Verification items for this drawing (mm, ordinates from the low corner). A direction names the side the tool comes from. Give positions to 0.01 mm unless a question says otherwise; leave off trailing zeros. Loops run counter-clockwise (first coordinate to the right, second up) from the corner with the lowest first, then second, coordinate; pieces in that order, holes last. Notation, with made-up numbers: M 10,-9.75 L 30,-9.75 A15 ccw 30,-4.75 Z; hole C -8,17 d7. An arc over 180 degrees is marked long. Use one line per item in the form item = value.
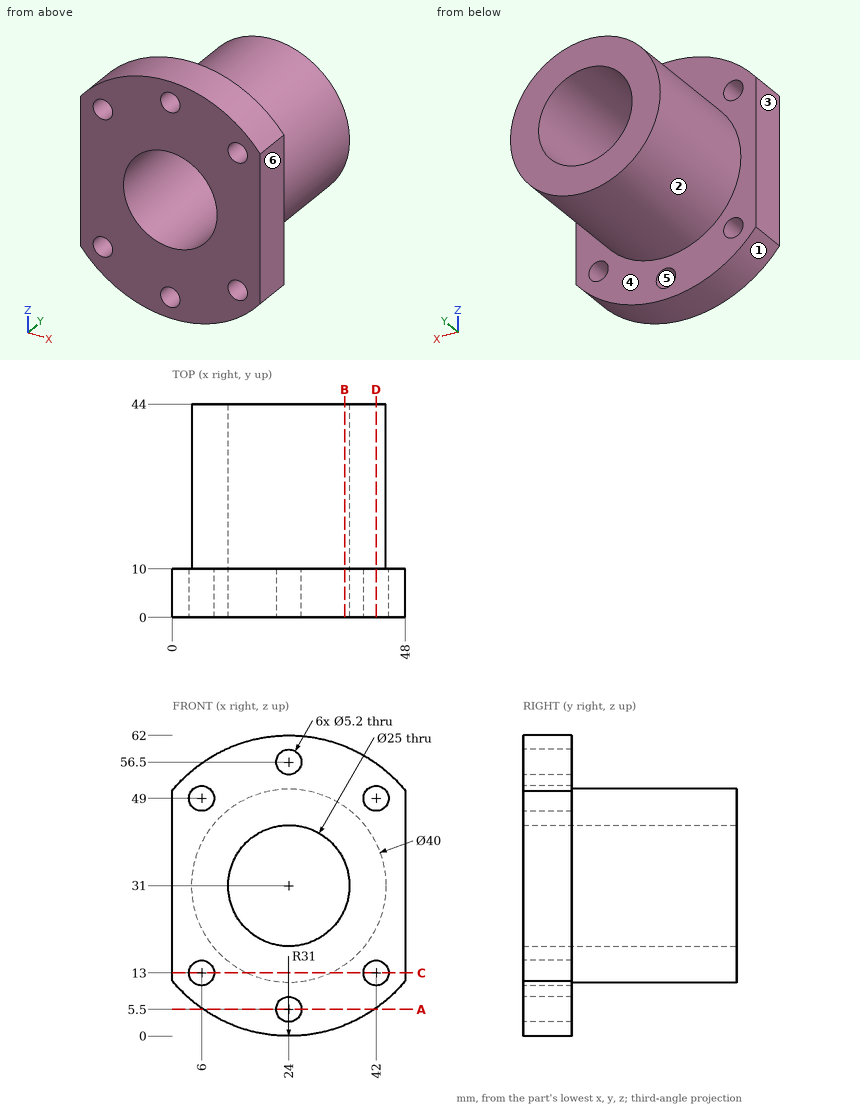
1) Section check C-C (z = 13). Record the cut outline in (x, y).
Evaluation:
outline = M 0,0 L 3.4,0 L 3.4,10 L 0,10 Z; M 8.6,0 L 39.4,0 L 39.4,10 L 32.72,10 L 32.72,44 L 15.28,44 L 15.28,10 L 8.6,10 Z; M 44.6,0 L 48,0 L 48,10 L 44.6,10 Z
2) Section check B-B (x = 35.5). Record the cut outline in (y, z), then the cut area to 3 significant figures.
Evaluation:
outline = M 0,2.21 L 10,2.21 L 10,14.64 L 44,14.64 L 44,26.1 L 0,26.1 Z; M 0,35.9 L 44,35.9 L 44,47.36 L 10,47.36 L 10,59.79 L 0,59.79 Z
area = 1,260 mm^2
3) Set-up check for the marked faces 1 and 2: record each of +Z, -Z, +X, -X, +Y, -Y from which the full face is reachable in a straight line by a thin tool's end or side.
Evaluation:
face_1 = -Z, +Y, -Y
face_2 = +Y
4) Depth check by flat-ended pin: pin 1 Ø4 at (x, z) = (37.5, 51) entering from +Y; pin 2 Ø5 at (x, y) = (37.5, 16.5) entering from +Z; pin 3 Ø12 at (y, z) = (22.5, 22) entering from +X. Enter the tip coordinate at first touch or a pass-through.
Evaluation:
pin_1 = 10
pin_2 = 47.7
pin_3 = 43.77
5) Scan lines: line 1 (X direction, y = 7.5, z = 49); line 2 (X direction, y = 18, z = 31); line 3 (Z direction, x = 24, y = 35). Record each from-to range of solid material in increasing order.
Evaluation:
line_1 = 0 to 3.4, 8.6 to 39.4, 44.6 to 48
line_2 = 4 to 11.5, 36.5 to 44
line_3 = 11 to 18.5, 43.5 to 51
6) Section check D-D (x = 42). Record the cut outline in (y, z).
Evaluation:
outline = M 0,5.76 L 10,5.76 L 10,10.4 L 0,10.4 Z; M 0,15.6 L 10,15.6 L 10,22.28 L 44,22.28 L 44,39.72 L 10,39.72 L 10,46.4 L 0,46.4 Z; M 0,51.6 L 10,51.6 L 10,56.24 L 0,56.24 Z
7) Release check for a two-part mould opening along X. For the marked faces 3, 4, 5 and 6 record: pulls with the +X half, pulls with the -X half, needs draft (parallel to the pull), parting line crosses it, or undercut.
Evaluation:
face_3 = pulls with the -X half
face_4 = needs draft
face_5 = undercut
face_6 = pulls with the +X half
8) Section check A-A (z = 5.5). Record the cut outline in (x, y).
Evaluation:
outline = M 6.37,0 L 21.4,0 L 21.4,10 L 6.37,10 Z; M 26.6,0 L 41.63,0 L 41.63,10 L 26.6,10 Z
